Can you work these out from the model? Positions are in its coordinate system, mm. Round coordinates to 2 decimals unless told otherwise and drop trailing zeros. Order: outer loops, then holes, each group sorted by start corner. A loop starts at its lowest first (then second) coordinate and runs counter-clockwise, first axis right, second up. Notation, with made-up numbers: M 81.25,15 L 98.25,15 A13 ccw 98.25,35 Z; hole C -17,72.5 d2. An arc over 180 degrees is marked long. Answer as a JSON object with one key per item and string values. Group by question number.
from build123d import *

# Parameters (mm, degrees)
SKETCH1_W            = 345.57
SKETCH1_H            = 56.55
BOSS_EXTRUDE1_DEPTH  = 6.35
SKETCH2_R            = 5
CUT_EXTRUDE1_DEPTH   = 10
LPATTERN1_COUNT      = 14
LPATTERN1_PITCH      = 21
LPATTERN1_COUNT_DIR2 = 3
LPATTERN1_PITCH_DIR2 = 15


with BuildPart() as part:
    # Sketch1 → Boss-Extrude1 (new body)
    with BuildSketch(Plane.XY):
        Rectangle(SKETCH1_W, SKETCH1_H)
    extrude(amount=BOSS_EXTRUDE1_DEPTH)

    # Sketch2 → Cut-Extrude1 (cut)
    with BuildSketch(Plane.XY.offset(6.35)):
        with Locations((-137.785, 15.775)):
            Circle(SKETCH2_R)
    cut_extrude1 = extrude(amount=-CUT_EXTRUDE1_DEPTH, mode=Mode.SUBTRACT)

    # LPattern1: Cut-Extrude1 14 × 3
    with Locations(*[(i * LPATTERN1_PITCH, -j * LPATTERN1_PITCH_DIR2, 0) for i in range(LPATTERN1_COUNT) for j in range(LPATTERN1_COUNT_DIR2) if (i, j) != (0, 0)]):
        add(cut_extrude1, mode=Mode.SUBTRACT)


solid = part.part
Item 1: Suppose I cut it at B-B, the plane z = 3.75. State how many separate pieces and enclosed holes the cut face has, and give its area (3 significant figures).
Item 2: If we mould it in two halves opening along X, with no side actions, what happens to faces 1 (the face through (-2, 28.275, 3)), 2 (the face through (172.785, 0, 3)), 3 (the face through (-15.75, -17.27, 3.22))? For each: +X half, -X half, draft (parallel to the pull), parting line (faces both ways), or undercut.
Item 3: I need wall thicknesses on line 1 (Y direction, x = 30.5, z = 5.75) (3 decimals); line 2 (Y direction, x = -72, z = 5.25) (3 decimals). Which ranges of each line are inside material? Lowest first, please.
Item 4: Suppose I cut it at A-A, the plane x = -115. Write out the boundary of the cut face in (y, z) (3 decimals), and give its area (3 significant figures).
Computed:
{
 "1": {"separate pieces": "1", "enclosed holes": "42", "area": "16,200 mm^2"},
 "2": {"face 1": "draft", "face 2": "+X half", "face 3": "undercut"},
 "3": {"line 1": "y = -28.275 to -19.217, -9.233 to -4.217, 5.767 to 10.783, 20.767 to 28.275", "line 2": "y = -28.275 to -18.378, -10.072 to -3.378, 4.928 to 11.622, 19.928 to 28.275"},
 "4": {"outline": "M -28.275,0 L -18.896,0 L -18.896,6.35 L -28.275,6.35 Z; M -9.554,0 L -3.896,0 L -3.896,6.35 L -9.554,6.35 Z; M 5.446,0 L 11.104,0 L 11.104,6.35 L 5.446,6.35 Z; M 20.446,0 L 28.275,0 L 28.275,6.35 L 20.446,6.35 Z", "area": "181 mm^2"}
}
